Build history of the part. All positions in model axes, mm. A direction names the side the tool comes from. Round coordinates to 2 decimals unless told otherwise and drop trailing zeros. Write each loop counter-clockwise with the first axis right and the second up, starting at its lowest first coordinate (ties: lowest second). Pieces come first, ordered by that corner, then holes. Notation, with made-up numbers: (32.5, -29.5) - (78.5, -29.5) arc R31 cw to (78.5, 5.5) - close; hole circle Ø11 at (-19, 28.25). An arc over 180 degrees is marked (long way). Write each question's results on one line, items separated by ' | '.
from build123d import *

# Parameters (mm, degrees)
SKETCH1_W               = 13
SKETCH1_H               = 4.5
BOSS_EXTRUDE1_DEPTH     = 0.375
BOSS_EXTRUDE2_DEPTH     = 1.25
BOSS_EXTRUDE3_DEPTH     = 2
SKETCH4_W               = 7
SKETCH4_H               = 0.5
CUT_EXTRUDE1_DEPTH      = 3.75
CUT_EXTRUDE2_DEPTH      = 7.95
CUT_EXTRUDE2_DEPTH_BACK = 7.95


with BuildPart() as part:
    # Sketch1 → Boss-Extrude1 (new body, symmetric)
    with BuildSketch(Plane.XY):
        Polygon((6.95, 2.25), (6.95, 2.75), (6.5, 2.75), (-6.5, 2.75), (-6.95, 2.75), (-6.95, 2.25), (-6.95, -2.25), (-6.95, -2.75), (-6.5, -2.75), (6.5, -2.75), (6.95, -2.75), (6.95, -2.25), align=None)
        Rectangle(SKETCH1_W, SKETCH1_H, mode=Mode.SUBTRACT)
        with BuildLine():
            Line((6.5, 1.875), (6.5, 2.25))
            Line((6.5, 2.25), (-6.5, 2.25))
            Line((-6.5, 2.25), (-6.5, 1.875))
            Line((-6.5, 1.875), (-6.5, 1))
            Line((-6.5, 1), (-6.5, -2.25))
            Line((-6.5, -2.25), (-2.834936491, -2.25))
            ThreePointArc((-2.834936491, -2.25), (-2.834936491, 0.25), (-5, 1.5))
            Line((-5, 1.5), (5, 1.5))
            ThreePointArc((5, 1.5), (2.834936491, 0.25), (2.834936491, -2.25))
            Line((2.834936491, -2.25), (6.5, -2.25))
            Line((6.5, -2.25), (6.5, 1))
            Line((6.5, 1), (6.5, 1.875))
        make_face()
        with BuildLine():
            Line((-2.834936491, -2.25), (2.834936491, -2.25))
            ThreePointArc((2.834936491, -2.25), (2.834936491, 0.25), (5, 1.5))
            Line((5, 1.5), (-5, 1.5))
            ThreePointArc((-5, 1.5), (-2.834936491, 0.25), (-2.834936491, -2.25))
        make_face()
    extrude(amount=BOSS_EXTRUDE1_DEPTH, both=True)

    # Sketch2 → Boss-Extrude2 (add)
    with BuildSketch(Plane(origin=(0, 0, -0.375), x_dir=(-1, 0, 0), z_dir=(0, 0, -1))):
        Polygon((-6.95, 2.25), (-6.95, -2.25), (-6.95, -2.75), (-6.5, -2.75), (6.5, -2.75), (6.95, -2.75), (6.95, -2.25), (6.95, 2.25), (6.95, 2.75), (6.5, 2.75), (-6.5, 2.75), (-6.95, 2.75), align=None)
        Polygon((-6.5, 1), (-6.5, 1.875), (-6.5, 2.25), (6.5, 2.25), (6.5, 1.875), (6.5, 1), (6.5, -2.25), (2.834936491, -2.25), (-2.834936491, -2.25), (-6.5, -2.25), align=None, mode=Mode.SUBTRACT)
    extrude(amount=BOSS_EXTRUDE2_DEPTH)

    # Sketch3 → Boss-Extrude3 (add)
    with BuildSketch(Plane(origin=(0, 0, -0.375), x_dir=(-1, 0, 0), z_dir=(0, 0, -1))):
        with BuildLine():
            ThreePointArc((-5, 1.5), (-2.834936491, 0.25), (-2.834936491, -2.25))
            Line((-2.834936491, -2.25), (2.834936491, -2.25))
            ThreePointArc((2.834936491, -2.25), (2.834936491, 0.25), (5, 1.5))
            Line((5, 1.5), (-5, 1.5))
        make_face()
    extrude(amount=BOSS_EXTRUDE3_DEPTH)

    # Sketch4 → Cut-Extrude1 (cut, through all)
    with BuildSketch(Plane(origin=(0, 0, -2.375), x_dir=(-1, 0, 0), z_dir=(0, 0, -1))):
        with Locations((0, 1.25)):
            Rectangle(SKETCH4_W, SKETCH4_H)
        with BuildLine():
            Line((3.5, 1.5), (3.5, 1))
            ThreePointArc((3.5, 1), (4.209430585, 1.371708245), (5, 1.5))
            Line((5, 1.5), (3.5, 1.5))
        make_face()
        with BuildLine():
            ThreePointArc((-5, 1.5), (-4.209430585, 1.371708245), (-3.5, 1))
            Line((-3.5, 1), (-3.5, 1.5))
            Line((-3.5, 1.5), (-5, 1.5))
        make_face()
    extrude(amount=-CUT_EXTRUDE1_DEPTH, mode=Mode.SUBTRACT)

    # Sketch5 → Cut-Extrude2 (cut, two sides)
    with BuildSketch(Plane(origin=(0, 0, 0), x_dir=(0, 0, -1), z_dir=(1, 0, 0))) as cut_extrude2_sk:
        with BuildLine():
            Line((3.875, 1.5), (0.375, 1.5))
            Line((0.375, 1.5), (0.375, 1))
            ThreePointArc((0.375, 1), (1.246708245, -1.790569415), (-1.125, -3.5))
            Line((-1.125, -3.5), (3.875, -3.5))
            Line((3.875, -3.5), (3.875, 1.5))
        make_face()
    extrude(amount=CUT_EXTRUDE2_DEPTH, mode=Mode.SUBTRACT)
    extrude(cut_extrude2_sk.sketch, amount=-CUT_EXTRUDE2_DEPTH_BACK, mode=Mode.SUBTRACT)


solid = part.part
(1) Slice it at C-C, the plane x = 0.75. Write the cut outline in (y, z) (3 decimals), and give its area (3 significant figures).
Worked answers:
outline: (-2.75, -0.66) arc R2.5 ccw to (1, -0.375) - (1, 0.375) - (-2.75, 0.375) - close; (1.5, -0.375) - (2.25, -0.375) - (2.25, -1.625) - (2.75, -1.625) - (2.75, 0.375) - (1.5, 0.375) - close | area: 7.13 mm2
(2) Flat gauge pin, fed straight in: pin 1 Ø1.5 at (x, y) = (0, -1.5) entering from -Z (3 decimals). Where does the tip first touch, or does it go through?
Worked answers:
pin 1: stops at z = -1.375
(3) Drill centre lines: probe 1 along X at (y, z) = (-0.9, -0.95); probe 2 along Y at (x, z) = (-2, 0.25); probe 3 along Y at (x, z) = (-3, -0.5). Where is each one in solid material? Low to high. Write a range as [from, to].
Worked answers:
probe 1: x = [-6.95, -6.5], [-2.5, 2.5], [6.5, 6.95] | probe 2: y = [-2.75, 1], [1.5, 2.75] | probe 3: y = [-2.75, -2.25], [0.5, 0.9], [2.25, 2.75]
(4) Slice it at A-A, the plane z = 0.2. Write the cut outline in (x, y), and give its area (3 significant figures).
Worked answers:
outline: (-6.95, -2.75) - (6.95, -2.75) - (6.95, 2.75) - (-6.95, 2.75) - close; hole (-5, 1.5) arc R2.5 cw to (-3.5, 1) - (3.5, 1) arc R2.5 cw to (5, 1.5) - close | area: 72.5 mm2
(5) Slice it at D-D, the plane x = -5.25. Write the cut outline in (y, z) (3 decimals), and give its area (3 significant figures).
Worked answers:
outline: (-2.75, -0.66) arc R2.5 ccw to (-2.25, -1.04) - (-2.25, -0.375) - (2.25, -0.375) - (2.25, -1.625) - (2.75, -1.625) - (2.75, 0.375) - (-2.75, 0.375) - close | area: 5.00 mm2
(6) Two-plate mould, pull along Y, no slides. Class faces 1 (the flat face through (0, 2.75, -1)), 2 (the cylindrical face through (2.5, -0.9, -0.8)), 3 (the flat face through (6.95, 0, 0)): released by +Y, released by -Y, zero draft, split by the parting line, or undercut.
Worked answers:
face 1: released by +Y | face 2: undercut | face 3: zero draft
(7) Tool access for faces 4 (the flat face through (6.5, -1, -1)), 5 (the flat face through (-6.95, 0, 0)): list every direction of +Z, -Z, +X, -X, +Y, -Y with a clear straight run to the whole face (end or side of a thin tool).
Worked answers:
face 4: -Z | face 5: +Z, -Z, -X, +Y, -Y
(8) Slice it at B-B, the plane y = 1.7. Write the cut outline in (x, z) (3 decimals).
Worked answers:
outline: (-6.95, -1.625) - (-6.5, -1.625) - (-6.5, -0.375) - (6.5, -0.375) - (6.5, -1.625) - (6.95, -1.625) - (6.95, 0.375) - (-6.95, 0.375) - close
